Check sheet for the modelled part. Datum: model origin and axes. Units: mm. Face numbers are marked on the shaded views. A direction names the side the tool comes from. Coordinates: 2 decimals unless noted, no trailing zeros. Loops run counter-clockwise (first coordinate to the right, second up) from the corner with the lowest first, then second, coordinate; pieces in that order, holes last.
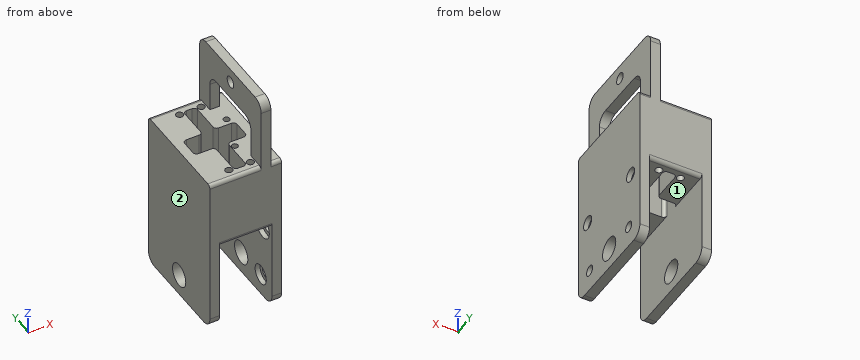
```python
from build123d import *

# Parameters (mm, degrees)
SKETCH1_W             = 20
SKETCH1_H             = 20
BOSS_EXTRUDE3_DEPTH   = 30
CUT_EXTRUDE11_REACH   = 39.417
SKETCH10_R            = 0.86
FILLET4_R             = 1
SKETCH12_W            = 2.7
SKETCH12_H            = 30
BOSS_EXTRUDE13_DEPTH  = 20
CUT_EXTRUDE13_REACH   = 47.706
SKETCH14_R            = 1.59
SKETCH14_W            = 11
SKETCH14_H            = 20
FILLET6_R             = 3
SKETCH16_W            = 2.7
SKETCH16_H            = 30
BOSS_EXTRUDE14_DEPTH  = 25
CUT_EXTRUDE14_REACH   = 51.237
SKETCH17_R            = 3.23
FILLET11_R            = 3
FILLET11_OF_MIRROR1_R = 3
FILLET12_R            = 1
CUT_EXTRUDE15_REACH   = 52.99
SKETCH18_R            = 1
CUT_EXTRUDE16_REACH   = 51.237
SKETCH20_R            = 1.98
SKETCH20_R_2          = 1.475
SKETCH22_R            = 2.725
SKETCH22_R_2          = 3.23
CUT_EXTRUDE17_DEPTH   = 1.35


with BuildPart() as part:
    # Sketch1 → Boss-Extrude3 (new body)
    with BuildSketch(Plane(origin=(0, 0, 0), x_dir=(1, 0, 0), z_dir=(0, 1, 0))):
        Rectangle(SKETCH1_W, SKETCH1_H)
    extrude(amount=BOSS_EXTRUDE3_DEPTH)

    # Sketch10 → Cut-Extrude11 (cut, up to next)
    with BuildSketch(Plane(origin=(0, 0, -10), x_dir=(-1, 0, 0), z_dir=(0, 0, -1)), mode=Mode.PRIVATE) as cut_extrude11_sk1:
        with Locations((-6, 19.86)):
            Circle(SKETCH10_R)
    cut_extrude11_tool1 = extrude(cut_extrude11_sk1.sketch, amount=-CUT_EXTRUDE11_REACH, mode=Mode.PRIVATE) & part.part
    # Sketch10 → Cut-Extrude11 (cut, up to next)
    with BuildSketch(Plane(origin=(0, 0, -10), x_dir=(-1, 0, 0), z_dir=(0, 0, -1)), mode=Mode.PRIVATE) as cut_extrude11_sk2:
        with Locations((-2.75, 10.14)):
            Circle(SKETCH10_R)
    cut_extrude11_tool2 = extrude(cut_extrude11_sk2.sketch, amount=-CUT_EXTRUDE11_REACH, mode=Mode.PRIVATE) & part.part
    # Sketch10 → Cut-Extrude11 (cut, up to next)
    with BuildSketch(Plane(origin=(0, 0, -10), x_dir=(-1, 0, 0), z_dir=(0, 0, -1)), mode=Mode.PRIVATE) as cut_extrude11_sk3:
        Polygon((-1.75, 27.5), (1.75, 27.5), (1.75, 18), (7.3, 18), (7.3, 12), (1.75, 12), (1.75, 2.5), (-1.75, 2.5), (-1.75, 12), (-7.3, 12), (-7.3, 18), (-1.75, 18), align=None)
    cut_extrude11_tool3 = extrude(cut_extrude11_sk3.sketch, amount=-CUT_EXTRUDE11_REACH, mode=Mode.PRIVATE) & part.part
    add(cut_extrude11_tool1.solids().sort_by_distance((6, 19.86, -10))[0], mode=Mode.SUBTRACT)
    add(cut_extrude11_tool2.solids().sort_by_distance((2.75, 10.14, -10))[0], mode=Mode.SUBTRACT)
    add(cut_extrude11_tool3.solids().sort_by_distance((0, 15, -10))[0], mode=Mode.SUBTRACT)

    # Fillet4
    fillet4_edges = [part.edges().sort_by_distance(p)[0] for p in [
        (-1.75, 2.5, 0),
        (1.75, 2.5, 0),
        (1.75, 12, 0),
        (7.3, 12, 0),
        (7.3, 18, 0),
        (1.75, 18, 0),
        (1.75, 27.5, 0),
        (-1.75, 27.5, 0),
        (-1.75, 18, 0),
        (-7.3, 18, 0),
        (-7.3, 12, 0),
        (-1.75, 12, 0),
    ]]
    fillet(fillet4_edges, radius=FILLET4_R)

    # Sketch12 → Boss-Extrude13 (add)
    with BuildSketch(Plane.XY.offset(10)):
        with Locations((5.65, 15)):
            Rectangle(SKETCH12_W, SKETCH12_H)
    extrude(amount=BOSS_EXTRUDE13_DEPTH)

    # Sketch14 → Cut-Extrude13 (cut, up to next)
    with BuildSketch(Plane(origin=(7, 0, 0), x_dir=(0, 0, -1), z_dir=(1, 0, 0)), mode=Mode.PRIVATE) as cut_extrude13_sk1:
        with Locations((-26, 15)):
            Circle(SKETCH14_R)
    cut_extrude13_tool1 = extrude(cut_extrude13_sk1.sketch, amount=-CUT_EXTRUDE13_REACH, mode=Mode.PRIVATE) & part.part
    # Sketch14 → Cut-Extrude13 (cut, up to next)
    with BuildSketch(Plane(origin=(7, 0, 0), x_dir=(0, 0, -1), z_dir=(1, 0, 0)), mode=Mode.PRIVATE) as cut_extrude13_sk2:
        with Locations((-15.5, 15)):
            Rectangle(SKETCH14_W, SKETCH14_H)
    cut_extrude13_tool2 = extrude(cut_extrude13_sk2.sketch, amount=-CUT_EXTRUDE13_REACH, mode=Mode.PRIVATE) & part.part
    add(cut_extrude13_tool1.solids().sort_by_distance((7, 15, 26))[0], mode=Mode.SUBTRACT)
    add(cut_extrude13_tool2.solids().sort_by_distance((7, 15, 15.5))[0], mode=Mode.SUBTRACT)

    # Fillet6
    fillet6_edges = [part.edges().sort_by_distance(p)[0] for p in [
        (5.65, 0, 30),
        (5.65, 30, 30),
        (5.65, 5, 21),
        (5.65, 25, 21),
    ]]
    fillet(fillet6_edges, radius=FILLET6_R)

    # Sketch16 → Boss-Extrude14 (add)
    with BuildSketch(Plane(origin=(0, 0, -10), x_dir=(-1, 0, 0), z_dir=(0, 0, -1))):
        with Locations((8.65, 15)):
            Rectangle(SKETCH16_W, SKETCH16_H)
    boss_extrude14 = extrude(amount=BOSS_EXTRUDE14_DEPTH)

    # Sketch17 → Cut-Extrude14 (cut, up to next)
    with BuildSketch(Plane(origin=(-7.3, 0, 0), x_dir=(0, 0, -1), z_dir=(1, 0, 0)), mode=Mode.PRIVATE) as cut_extrude14_sk1:
        with Locations((29, 15)):
            Circle(SKETCH17_R)
    cut_extrude14_tool1 = extrude(cut_extrude14_sk1.sketch, amount=-CUT_EXTRUDE14_REACH, mode=Mode.PRIVATE) & part.part
    cut_extrude14 = cut_extrude14_tool1.solids().sort_by_distance((-7.3, 15, -29))[0]
    add(cut_extrude14, mode=Mode.SUBTRACT)

    # Fillet11
    fillet11_edges = [part.edges().sort_by_distance(p)[0] for p in [
        (-8.65, 30, -35),
        (-8.65, 0, -35),
    ]]
    fillet(fillet11_edges, radius=FILLET11_R)

    # Mirror1: Boss-Extrude14, Cut-Extrude14 across plane
    add(boss_extrude14.mirror(Plane(origin=(0, 0, 0), x_dir=(0, 0, 1), z_dir=(1, 0, 0))))
    add(cut_extrude14.mirror(Plane(origin=(0, 0, 0), x_dir=(0, 0, 1), z_dir=(1, 0, 0))), mode=Mode.SUBTRACT)

    # Fillet11 of Mirror1
    fillet11_of_mirror1_edges = [part.edges().sort_by_distance(p)[0] for p in [
        (8.65, 30, -35),
        (8.65, 0, -35),
    ]]
    fillet(fillet11_of_mirror1_edges, radius=FILLET11_OF_MIRROR1_R)

    # Fillet12
    fillet12_edges = [part.edges().sort_by_distance(p)[0] for p in [
        (8.5, 0, 10),
        (8.5, 30, 10),
        (0, 0, -10),
        (0, 30, -10),
        (-2.85, 30, 10),
        (-2.85, 0, 10),
    ]]
    fillet(fillet12_edges, radius=FILLET12_R)

    # Sketch18 → Cut-Extrude15 (cut, up to next)
    with BuildSketch(Plane(origin=(0, 0, -10), x_dir=(-1, 0, 0), z_dir=(0, 0, -1)), mode=Mode.PRIVATE) as cut_extrude15_sk1:
        with Locations((-3, 27)):
            Circle(SKETCH18_R)
    cut_extrude15_tool1 = extrude(cut_extrude15_sk1.sketch, amount=-CUT_EXTRUDE15_REACH, mode=Mode.PRIVATE) & part.part
    # Sketch18 → Cut-Extrude15 (cut, up to next)
    with BuildSketch(Plane(origin=(0, 0, -10), x_dir=(-1, 0, 0), z_dir=(0, 0, -1)), mode=Mode.PRIVATE) as cut_extrude15_sk2:
        with Locations((3, 3)):
            Circle(SKETCH18_R)
    cut_extrude15_tool2 = extrude(cut_extrude15_sk2.sketch, amount=-CUT_EXTRUDE15_REACH, mode=Mode.PRIVATE) & part.part
    cut_extrude15_1 = cut_extrude15_tool1.solids().sort_by_distance((3, 27, -10))[0]
    add(cut_extrude15_1, mode=Mode.SUBTRACT)
    cut_extrude15_2 = cut_extrude15_tool2.solids().sort_by_distance((-3, 3, -10))[0]
    add(cut_extrude15_2, mode=Mode.SUBTRACT)
    cut_extrude15 = cut_extrude15_1 + cut_extrude15_2  # Cut-Extrude15 as one shape, for the pattern or mirror that repeats it

    # Mirror2: Cut-Extrude15 across plane
    add(cut_extrude15.mirror(Plane(origin=(0, 0, 0), x_dir=(0, 0, 1), z_dir=(1, 0, 0))), mode=Mode.SUBTRACT)

    # Sketch20 → Cut-Extrude16 (cut, up to next)
    with BuildSketch(Plane.ZY.offset(7.3), mode=Mode.PRIVATE) as cut_extrude16_sk1:
        with Locations((-13.25, 25.48)):
            Circle(SKETCH20_R)
    cut_extrude16_tool1 = extrude(cut_extrude16_sk1.sketch, amount=-CUT_EXTRUDE16_REACH, mode=Mode.PRIVATE) & part.part
    # Sketch20 → Cut-Extrude16 (cut, up to next)
    with BuildSketch(Plane.ZY.offset(7.3), mode=Mode.PRIVATE) as cut_extrude16_sk2:
        with Locations((-13.25, 4.52)):
            Circle(SKETCH20_R)
    cut_extrude16_tool2 = extrude(cut_extrude16_sk2.sketch, amount=-CUT_EXTRUDE16_REACH, mode=Mode.PRIVATE) & part.part
    # Sketch20 → Cut-Extrude16 (cut, up to next)
    with BuildSketch(Plane.ZY.offset(7.3), mode=Mode.PRIVATE) as cut_extrude16_sk3:
        with Locations((-29, 5.48)):
            Circle(SKETCH20_R_2)
    cut_extrude16_tool3 = extrude(cut_extrude16_sk3.sketch, amount=-CUT_EXTRUDE16_REACH, mode=Mode.PRIVATE) & part.part
    # Sketch20 → Cut-Extrude16 (cut, up to next)
    with BuildSketch(Plane.ZY.offset(7.3), mode=Mode.PRIVATE) as cut_extrude16_sk4:
        with Locations((-29, 24.52)):
            Circle(SKETCH20_R_2)
    cut_extrude16_tool4 = extrude(cut_extrude16_sk4.sketch, amount=-CUT_EXTRUDE16_REACH, mode=Mode.PRIVATE) & part.part
    add(cut_extrude16_tool1.solids().sort_by_distance((-7.3, 25.48, -13.25))[0], mode=Mode.SUBTRACT)
    add(cut_extrude16_tool2.solids().sort_by_distance((-7.3, 4.52, -13.25))[0], mode=Mode.SUBTRACT)
    add(cut_extrude16_tool3.solids().sort_by_distance((-7.3, 5.48, -29))[0], mode=Mode.SUBTRACT)
    add(cut_extrude16_tool4.solids().sort_by_distance((-7.3, 24.52, -29))[0], mode=Mode.SUBTRACT)

    # Sketch22 → Cut-Extrude17 (cut)
    with BuildSketch(Plane.ZY.offset(-7.3)):
        with Locations(Location((-29, 24.52, 0), (0, 0, 270))):
            Circle(SKETCH22_R)
        with Locations(Location((-13.25, 25.48, 0), (0, 0, 270))):
            Circle(SKETCH22_R_2)
        with Locations(Location((-13.25, 4.52, 0), (0, 0, 270))):
            Circle(SKETCH22_R_2)
        with Locations(Location((-29, 5.48, 0), (0, 0, 270))):
            Circle(SKETCH22_R)
    extrude(amount=-CUT_EXTRUDE17_DEPTH, mode=Mode.SUBTRACT)


solid = part.part
```
1) Section check A-A on z = 14.5. Enter the section's corners in (x, y).
Answer sheet:
outline: (4.3, 0) - (7, 0) - (7, 5) - (4.3, 5) - close; (4.3, 25) - (7, 25) - (7, 30) - (4.3, 30) - close
2) Section check C-C on z = -13.25. Enter the section's corners in (x, y), plus the area to 3 significant figures.
Answer sheet:
outline: (-10, 0) - (-7.3, 0) - (-7.3, 30) - (-10, 30) - close; (7.3, 0) - (10, 0) - (10, 2.54) - (8.65, 2.54) - (8.65, 1.29) - (7.3, 1.29) - close; (7.3, 7.75) - (8.65, 7.75) - (8.65, 6.5) - (10, 6.5) - (10, 23.5) - (8.65, 23.5) - (8.65, 22.25) - (7.3, 22.25) - close; (7.3, 28.71) - (8.65, 28.71) - (8.65, 27.46) - (10, 27.46) - (10, 30) - (7.3, 30) - close
area: 134 mm2
3) Set-up check for the marked faces 1 and 2: record each of +Z, -Z, +X, -X, +Y, -Y from which the full face is reachable in a straight line by a thin tool's end or side.
Answer sheet:
face 1: -Z, +Y, -Y
face 2: +Z, -Z, -X, +Y, -Y
4) Scan lines: line 1 (Y direction, x = 9.1, z = -13.25); line 2 (X direction, y = 10, z = 0.5); line 3 (X direction, y = 5.75, z = -15). Record each from-to range of solid material in increasing order.
Answer sheet:
line 1: y = 0 to 2.54, 6.5 to 23.5, 27.46 to 30
line 2: x = -10 to -1.75, 1.75 to 1.9, 3.6 to 10
line 3: x = -10 to -7.3, 8.65 to 10
5) Depth check by flat-ended pin: pin 1 (3 mm diameter, centred on x = -5, y = 5.5, fed in from -Z); pin 2 (6 mm diameter, centred on y = 15, z = -29, fed in from -X); pin 3 (1.4 mm diameter, centred on x = 6, y = 19.86, fed in from -Z); pin 4 (10 mm diameter, centred on x = -3.5, y = 17.5, fed in from +Z). Enter the tip coordinate at first touch or a pass-through.
Answer sheet:
pin 1: stops at z = -10
pin 2: passes through
pin 3: stops at z = 21
pin 4: stops at z = 10
6) Section check B-B on z = -3. Give the number of separate pieces and of enclosed holes in the cut face, plus the area to 3 significant figures.
Answer sheet:
separate pieces: 1
enclosed holes: 7
area: 430 mm2
